from build123d import *

# Parameters (mm, degrees)
SKETCH1_R           = 1.7000000000000015
SKETCH1_R_2         = 1.1249999999999982
BOSS_EXTRUDE1_DEPTH = 30
CUT_EXTRUDE1_DEPTH  = 3.5
CUT_EXTRUDE2_DEPTH  = 3.5
FILLET1_R           = 4
SKETCH6_W           = 16.8927871134671
SKETCH6_H           = 14
CUT_EXTRUDE3_DEPTH  = 96.70345562354154
CUT_EXTRUDE4_DEPTH  = 3
FILLET2_R           = 3
FILLET3_R           = 3
CUT_EXTRUDE7_DEPTH  = 10
FILLET4_R           = 3
FILLET5_R           = 3


with BuildPart() as part:
    # Sketch1 → Boss-Extrude1 (new body)
    with BuildSketch(Plane(origin=(0, 0, 0), x_dir=(1, 0, 0), z_dir=(0, 1, 0))):
        with BuildLine():
            Line((-67.41726719036473, 89.75450030463905), (-64.96978375504433, 89.75450030463905))
            Line((-64.96978375504433, 89.75450030463905), (-53.48663897336089, 66.16198945077305))
            ThreePointArc((-53.48663897336089, 66.16198945077305), (-53.65304900524508, 63.02325116523408), (-56.40241603973214, 61.499981250381275))
            Line((-56.40241603973214, 61.499981250381275), (-67.41726719036473, 61.499981250381275))
            Line((-67.41726719036473, 61.499981250381275), (-67.41726719036473, 89.75450030463905))
        make_face()
        with Locations(Location((-63.06696708972735, 65.27360292976877, 0), (0, 0, 270))):
            Circle(SKETCH1_R, mode=Mode.SUBTRACT)
        with Locations(Location((-56.40241603973214, 64.74279797888421, 0), (0, 0, 270))):
            Circle(SKETCH1_R_2, mode=Mode.SUBTRACT)
    extrude(amount=BOSS_EXTRUDE1_DEPTH)

    # Sketch4 → Cut-Extrude1 (cut)
    with BuildSketch(Plane(origin=(0, 0, 0), x_dir=(-1, 0, 0), z_dir=(0, -1, 0))):
        Polygon((56.36085478477071, 72.24701778462617), (67.25774228220871, 68.66563773680312), (67.56486364186908, 68.5646989769961), (68.07491191484384, 60.66505530671413), (50.67511099214203, 61.303323516745735), (50.323559595932146, 66.74816258197976), align=None)
    extrude(amount=-CUT_EXTRUDE1_DEPTH, mode=Mode.SUBTRACT)

    # Sketch5 → Cut-Extrude2 (cut)
    with BuildSketch(Plane(origin=(0, 30, 0), x_dir=(1, 0, 0), z_dir=(0, 1, 0))):
        Polygon((-56.36085478477071, 72.24701778462617), (-67.25774228220871, 68.66563773680312), (-69.83403727288335, 67.81891049665515), (-69.83403727288335, 60.473378762572615), (-51.53143062922566, 60.473378762572615), (-50.58101521609465, 66.57187766349658), align=None)
    extrude(amount=-CUT_EXTRUDE2_DEPTH, mode=Mode.SUBTRACT)

    # Fillet1
    fillet1_edges = [part.edges().sort_by_distance(p)[0] for p in [
        (-67.41726719036473, 15, -61.499981250381275),
    ]]
    fillet(fillet1_edges, radius=FILLET1_R)

    # Sketch6 → Cut-Extrude3 (cut, through all)
    with BuildSketch(Plane.ZY.offset(67.41726719036473)):
        with Locations((-65.05358769364771, 16.5)):
            Rectangle(SKETCH6_W, SKETCH6_H)
    extrude(amount=-CUT_EXTRUDE3_DEPTH, mode=Mode.SUBTRACT)

    # Sketch7 → Cut-Extrude4 (cut)
    with BuildSketch(Plane(origin=(0, 3.5, 0), x_dir=(-1, 0, 0), z_dir=(0, -1, 0))):
        Polygon((56.43632253896984, 72.22221449018052), (53.48663897336088, 66.16198945077305), (50.72300756793861, 60.4840148917036), (56.40241603973214, 61.499981250381275), (59.909841615048435, 61.499981250381275), (59.909841615048435, 70.20099101348265), (59.909841615048435, 71.08060484084474), align=None)
    extrude(amount=-CUT_EXTRUDE4_DEPTH, mode=Mode.SUBTRACT)

    # Fillet2
    fillet2_edges = [part.edges().sort_by_distance(p)[0] for p in [
        (-59.909841615048435, 5, -61.499981250381275),
    ]]
    fillet(fillet2_edges, radius=FILLET2_R)

    # Fillet3
    fillet3_edges = [part.edges().sort_by_distance(p)[0] for p in [
        (-59.909841615048435, 5, -71.08060484084474),
    ]]
    fillet(fillet3_edges, radius=FILLET3_R)

    # Sketch8 → Cut-Extrude7 (cut)
    with BuildSketch(Plane(origin=(0, 26.5, 0), x_dir=(1, 0, 0), z_dir=(0, 1, 0))):
        Polygon((-59.61138736288163, 71.17869506194207), (-60.80258919639462, 70.78719368317894), (-58.46431809995156, 61.499981250381275), (-56.120645243524336, 59.6371858222966), (-50.85616204416965, 63.63562557653779), (-56.436322538969726, 72.22221449018029), align=None)
    extrude(amount=-CUT_EXTRUDE7_DEPTH, mode=Mode.SUBTRACT)

    # Fillet4
    fillet4_edges = [part.edges().sort_by_distance(p)[0] for p in [
        (-58.46431809995156, 25, -61.499981250381275),
    ]]
    fillet(fillet4_edges, radius=FILLET4_R)

    # Fillet5
    fillet5_edges = [part.edges().sort_by_distance(p)[0] for p in [
        (-60.80258919639462, 25, -70.78719368317894),
    ]]
    fillet(fillet5_edges, radius=FILLET5_R)


solid = part.part
Input: part model. Units: mm. Frame: model coordinates. A direction names the side the tool comes from. Give positions to 0.01 mm unless a question says otherwise; leave off trailing zeros. Order: outer loops, then holes, each group sorted by start corner. A loop starts at its lowest first (then second) coordinate and runs counter-clockwise, first axis right, second up. Notation, with made-up numbers: (-39, 75.25) - (-28, 75.25) arc R31 cw to (-28, 105.25) - close; hole circle Ø2 at (-10.5, 44). An arc over 180 degrees is marked (long way). Write each question's results on one line, items separated by ' | '.
Item 1: Section C-C (y = 16.75). Return loops of the section in (x, z), and give its area (3 significant figures).
A:
outline: (-67.42, -89.75) - (-64.97, -89.75) - (-57.06, -73.5) - (-67.42, -73.5) - close | area: 104 mm^2
Item 2: Access query for faces 5 (the cylindrical face through (-59.854, 24.979, -70.229)), 6 (the flat face through (-63, 23.5, -69)), 7 (the flat face through (-62.004, 1.76, -70.392)). Directions: +Z, -Z, +X, -X, +Y, -Y. A direction counts if a zero-diameter tool reaches every point of the face in a straight line with its end or side. Return the directions, or none.
A:
face 5: +X, +Y | face 6: +Z, +X, -X | face 7: +Z, +X, -Y
Item 3: Material intervals for line 1 along Y through (x, z) = (-64, -63.75); line 2 along Y through (x, z) = (-64, -72.5); line 3 along Y through (x, z) = (-57, -71.5), sorted ascending.
A:
line 1: y = 3.5 to 9.5, 23.5 to 26.5 | line 2: y = 0 to 9.5, 23.5 to 30 | line 3: y = 6.5 to 9.5
Item 4: Section A-A (z = -70.5). Return loops of the section in (x, y).
A:
outline: (-67.42, 0) - (-61.68, 0) - (-61.68, 3.5) - (-59.45, 3.5) - (-59.45, 6.5) - (-55.6, 6.5) - (-55.6, 9.5) - (-67.42, 9.5) - close; (-67.42, 23.5) - (-59.69, 23.5) - (-59.69, 26.5) - (-61.68, 26.5) - (-61.68, 30) - (-67.42, 30) - close
Item 5: Contact query for flat-ended pins moving along their axis: pin 1 Ø3.5 at (x, z) = (-57, -68.5) entering from +Y; pin 2 Ø3 at (x, z) = (-66, -68) entering from -Y; pin 3 Ø4 at (y, z) = (10.5, -77) entering from +X; pin 4 Ø3 at (y, z) = (16.5, -77) entering from +X. Output: stop coordinate, or through.
A:
pin 1: stops at y = 9.5 | pin 2: stops at y = 0 | pin 3: stops at x = -57.79 | pin 4: stops at x = -58.03
Item 6: Section B-B (y = 5.25). Return loops of the section in (x, z), and give its area (3 significant figures).
A:
outline: (-67.42, -89.75) - (-64.97, -89.75) - (-56.44, -72.22) - (-57.85, -71.76) arc R3 cw to (-59.91, -68.91) - (-59.91, -64.5) arc R3 ccw to (-62.91, -61.5) - (-63.42, -61.5) arc R4 ccw to (-67.42, -65.5) - close; hole circle Ø3.4 at (-63.07, -65.27) | area: 187 mm^2
Item 7: Section D-D (z = -87.5). Return loops of the section in (x, y), and give its area (3 significant figures).
A:
outline: (-67.42, 0) - (-63.87, 0) - (-63.87, 30) - (-67.42, 30) - close | area: 106 mm^2
Item 8: Draft query along X for faces 1 (the flat face through (-66, 15, -89.755)), 2 (the cylindrical face through (-63.718, 24.979, -63.703)), 3 (the cylindrical face through (-57.5, 7.98, -64.99)), 4 (the cylindrical face through (-59.324, 5.021, -70.689)). Return one class per face: released by +X, released by -X, zero draft, split by the parting line, or undercut.
A:
face 1: zero draft | face 2: undercut | face 3: undercut | face 4: released by +X
